Design review of the part shown in the three views and the two pictorial views. Dimensions are in mm from the part's minimum x, y and z. A direction names the side the tool comes from. Round coordinates to 2 decimals unless told otherwise and drop trailing zeros. Order: outer loops, then holes, each group sorted by start corner. A loop starts at its lowest first (then second) coordinate and runs counter-clockwise, first axis right, second up. Notation, with made-up numbers: M 63.25,-10.5 L 81.25,-10.5 A11 ccw 81.25,-5.5 Z; hole C 52,-16.75 d7. An arc over 180 degrees is marked long. Use a Markdown table: item, result. Add a question column.
(1) The part is to be moulded in two halves that separate along Z. For the marked faces 4, 5 and 6, say which applies: released by +Z, released by -Z, zero draft, split by the parting line, or undercut.
(2) Take a section at C-C (z = 1.5). Write out the cut boundary in (x, y), then the cut area to 3 significant figures.
(3) Take a section at A-A (x = 15). Count the separate pieces of the cut face and the enclosed holes in it, then the cut area to 3 significant figures.
(4) For pin 1 (3 mm diameter, centred on x = 15, y = 4, fed in from +Z); pin 2 (3 mm diameter, centred on x = 17.5, z = 7.5, fed in from +Y); pin 3 (4.5 mm diameter, centred on x = 15, y = 5.144, fed in from +Z); pin 4 (4.5 mm diameter, centred on x = 14.5, y = 44.5, fed in from +Z), all flat-tipped, find the tip position at first contact; note any pin that passes through.
(5) Take a section at D-D (x = 4.5). Write out the cut boundary in (y, z).
(6) To check wall thickness, follow probe 1 along Y at (x, z) = (15, 1.4); probe 2 along Y at (x, z) = (15, 4.2); probe 3 along Z at (x, y) = (14.5, 16.5). State the ranges of each line that lie inside material, in increasing order. Write a range as from..to.
(7) Take a section at B-B (z = 4). Write out the cut boundary in (x, y), then the cut area to 3 significant figures.
(8) Machinability: for the marked faces 1, 2 and 3, which of the approach directions +Z, -Z, +X, -X, +Y, -Y give a long, thin tool a straight path to every point of the face, cutting with its end or side? Answer none if there is none.
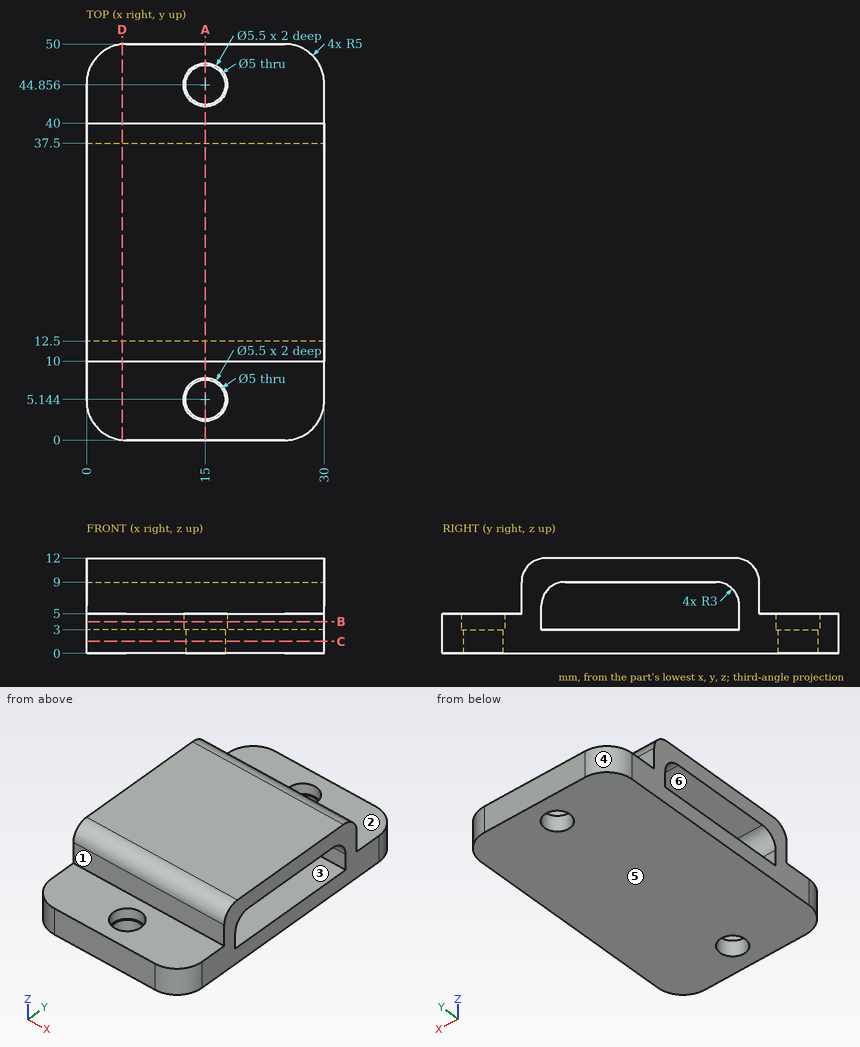
Verdict:
| question | item | result |
|---|---|---|
| 1 | face 4 | zero draft |
| 1 | face 5 | released by -Z |
| 1 | face 6 | undercut |
| 2 | outline | M 0,5 A5 ccw 5,0 L 25,0 A5 ccw 30,5 L 30,45 A5 ccw 25,50 L 5,50 A5 ccw 0,45 Z; hole C 15,5.14 d5; hole C 15,44.86 d5 |
| 2 | area | 1,440 mm^2 |
| 3 | separate pieces | 3 |
| 3 | enclosed holes | 1 |
| 3 | area | 258 mm^2 |
| 4 | pin 1 | stops at z = 3 |
| 4 | pin 2 | stops at y = 40 |
| 4 | pin 3 | passes through |
| 4 | pin 4 | stops at z = 5 |
| 5 | outline | M 0.03,0 L 49.97,0 L 49.97,5 L 40,5 L 40,9 A3 ccw 37,12 L 13,12 A3 ccw 10,9 L 10,5 L 0.03,5 Z; hole M 12.5,3 L 37.5,3 L 37.5,6 A3 ccw 34.5,9 L 15.5,9 A3 ccw 12.5,6 Z |
| 6 | probe 1 | y = 0..2.64, 7.64..42.36, 47.36..50 |
| 6 | probe 2 | y = 0..2.39, 7.89..12.5, 37.5..42.11, 47.61..50 |
| 6 | probe 3 | z = 0..3, 9..12 |
| 7 | outline | M 0,5 A5 ccw 5,0 L 25,0 A5 ccw 30,5 L 30,12.5 L 0,12.5 Z; M 0,37.5 L 30,37.5 L 30,45 A5 ccw 25,50 L 5,50 A5 ccw 0,45 Z; hole C 15,5.14 d5.5; hole C 15,44.86 d5.5 |
| 7 | area | 681 mm^2 |
| 8 | face 1 | +Z, +X, -X, -Y |
| 8 | face 2 | +Z, +X, -X, +Y |
| 8 | face 3 | +X, -X |
